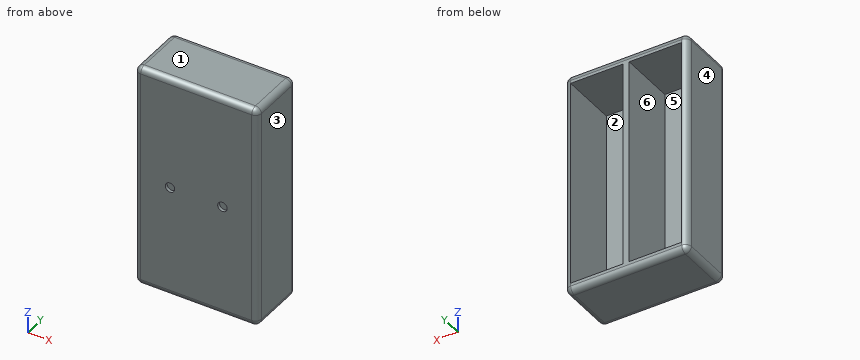
```python
from build123d import *

# Parameters (mm, degrees)
SKETCH_1_W          = 41.5
SKETCH_1_H          = 76
EXTRUDE_1_DEPTH     = 20
SKETCH_2_W          = 17.75
SKETCH_2_H          = 70
CUT_EXTRUDE_1_DEPTH = 19
SKETCH_3_R          = 1.6
CUT_EXTRUDE_2_DEPTH = 19
FILLET_1_R          = 2


with BuildPart() as part:
    # 草图1 → 凸台-拉伸1 (new body)
    with BuildSketch(Plane(origin=(0, 0, 0), x_dir=(1, 0, 0), z_dir=(0, 1, 0))):
        Rectangle(SKETCH_1_W, SKETCH_1_H)
    extrude(amount=EXTRUDE_1_DEPTH)

    # 草图2 → 切除-拉伸1 (cut)
    with BuildSketch(Plane(origin=(0, 20, 0), x_dir=(1, 0, 0), z_dir=(0, 1, 0))):
        with Locations((-9.875, 0)):
            Rectangle(SKETCH_2_W, SKETCH_2_H)
        with Locations((9.875, 0)):
            Rectangle(SKETCH_2_W, SKETCH_2_H)
    extrude(amount=-CUT_EXTRUDE_1_DEPTH, mode=Mode.SUBTRACT)

    # 草图3 → 切除-拉伸2 (cut)
    with BuildSketch(Plane(origin=(0, 1, 0), x_dir=(1, 0, 0), z_dir=(0, 1, 0))):
        with Locations(Location((-8.85, 0, 0), (0, 0, 270))):
            Circle(SKETCH_3_R)
        with Locations(Location((8.85, 0, 0), (0, 0, 90))):
            Circle(SKETCH_3_R)
    extrude(amount=-CUT_EXTRUDE_2_DEPTH, mode=Mode.SUBTRACT)

    # 圆角1
    fillet_1_edges = [part.edges().sort_by_distance(p)[0] for p in [
        (-20.75, 20, 0),
        (0, 20, 38),
        (20.75, 20, 0),
        (0, 0, 38),
        (-20.75, 0, 0),
        (0, 0, -38),
        (20.75, 0, 0),
        (20.75, 10, 38),
        (-20.75, 10, 38),
        (-20.75, 10, -38),
        (20.75, 10, -38),
        (0, 20, -38),
    ]]
    fillet(fillet_1_edges, radius=FILLET_1_R - 0.0001)  # a hair under: the kernel refuses the full size


solid = part.part
```
Input: part model. Units: mm. Frame: model coordinates. Face numbers are marked on the shaded views. A direction names the side the tool comes from. Give positions to 0.01 mm unless a question says otherwise; leave off trailing zeros. Order: outer loops, then holes, each group sorted by start corner. A loop starts at its lowest first (then second) coordinate and runs counter-clockwise, first axis right, second up. Notation, with made-up numbers: M 82,10.25 L 121,10.25 A24 ccw 121,34.25 Z; hole C 64.5,83.25 d9. An arc over 180 degrees is marked long. Return JSON: item names as keys, results as strings.
1) Section query B-B on z = 0. Count the separate pieces of the cut face and the enclosed holes in it, and give its area (3 significant figures).
Taken from the geometry:
{"separate pieces": "3", "enclosed holes": "0", "area": "146 mm2"}
2) Section query A-A on x = -8.85. Output: boundary loops of the cut face in (y, z).
Taken from the geometry:
{"outline": "M 0,-36 A2 ccw 2,-38 L 18,-38 A2 ccw 20,-36 L 20,-35 L 1,-35 L 1,-1.6 L 0,-1.6 Z; M 0,1.6 L 1,1.6 L 1,35 L 20,35 L 20,36 A2 ccw 18,38 L 2,38 A2 ccw 0,36 Z"}
3) Line query: L1, parallel to X at y = 3.5, z = -28.5; L2, parallel to Z at x = -14.5, y = 6.75; L3, parallel to X at y = 0.35, z = 0. Output: solid intervals per line, ascending. Write a range as [from, to].
Taken from the geometry:
{"L1": "x = [-20.75, -18.75], [-1, 1], [18.75, 20.75]", "L2": "z = [-38, -35], [35, 38]", "L3": "x = [-19.88, -10.45], [-7.25, 7.25], [10.45, 19.88]"}
4) Contact query for flat-ended pins moving along their axis: pin 1 (3 mm diameter, centred on x = -8.85, z = 0, fed in from -Y); pin 2 (19.5 mm diameter, centred on x = 11.5, z = 7.5, fed in from +Y); pin 3 (5.5 mm diameter, centred on x = -7, z = -5.5, fed in from +Y). Output: stop coordinate, or through.
Taken from the geometry:
{"pin 1": "passes through", "pin 2": "stops at y = 20", "pin 3": "stops at y = 1"}
5) Access query for the marked faces 1 and 2. Directions: +Z, -Z, +X, -X, +Y, -Y. A direction counts if a zero-diameter tool reaches every point of the face in a straight line with its end or side. Return the directions, or none.
Taken from the geometry:
{"face 1": "+Z, +X, -X, +Y, -Y", "face 2": "+Y"}
6) Mould query, pull axis X, two halves, no side actions, for the marked faces 3, 4, 5 and 6. Classes: released by +X, released by -X, zero draft, split by the parting line, or undercut.
Taken from the geometry:
{"face 3": "released by +X", "face 4": "released by -X", "face 5": "undercut", "face 6": "undercut"}
7) Section query C-C on y = 5. Output: boundary loops of the cut face in (x, z).
Taken from the geometry:
{"outline": "M -20.75,-36 A2 ccw -18.75,-38 L 18.75,-38 A2 ccw 20.75,-36 L 20.75,36 A2 ccw 18.75,38 L -18.75,38 A2 ccw -20.75,36 Z; hole M -18.75,-35 L -1,-35 L -1,35 L -18.75,35 Z; hole M 1,-35 L 18.75,-35 L 18.75,35 L 1,35 Z"}
